Could you check a few things on this model? Use its own coordinates, in mm. Face numbers are marked on the shaded views. A direction names the side the tool comes from. Give positions to 0.01 mm unless a question says otherwise; leave off trailing zeros. Order: outer loops, then holes, each group sorted by start corner. A loop starts at its lowest first (then second) coordinate and runs counter-clockwise, first axis right, second up.
from build123d import *

# Parameters (mm, degrees)
F1_DEPTH  = 12.6
F2_R      = 6
F3_DEPTH  = 16
F4_R      = 3.85
F5_DEPTH  = 5.8
F6_R      = 4.35
F7_DEPTH  = 3.6
F8_R      = 2
F9_R      = 1.5
F10_W     = 1
F10_H     = 5
F11_DEPTH = 5
F12_R     = 1.2
F13_DEPTH = 10.501


with BuildPart() as f1:
    # F0 (on Top) → F1 (new body)
    with BuildSketch(Plane.XY):
        with BuildLine():
            Line((-6.15, -6.5), (12.65, -6.5))
            Line((12.65, -6.5), (12.65, 6.5))
            Line((12.65, 6.5), (-6.15, 6.5))
            ThreePointArc((-6.15, 6.5), (-10.746194, 4.596194), (-12.65, 0))
            ThreePointArc((-12.65, 0), (-10.746194, -4.596194), (-6.15, -6.5))
        make_face()
    extrude(amount=-F1_DEPTH)

    # F2 (on Top) → F3 (join)
    with BuildSketch(Plane.XY):
        Circle(F2_R)
    extrude(amount=F3_DEPTH)

    # F4 (on face) → F5 (join)
    with BuildSketch(Plane.XY.offset(16)):
        Circle(F4_R)
    extrude(amount=F5_DEPTH)

    # F6 (on face) → F7 (join)
    with BuildSketch(Plane.XY.offset(21.8)):
        Circle(F6_R)
    extrude(amount=F7_DEPTH)

    # F8
    f8_edges = [f1.edges().sort_by_distance(p)[0] for p in [
        (-4.35, 0, 25.4),
    ]]
    fillet(f8_edges, radius=F8_R)

    # F9
    f9_edges = [f1.edges().sort_by_distance(p)[0] for p in [
        (3.25, -6.5, -12.6),
        (12.65, 0, -12.6),
        (3.25, 6.5, -12.6),
        (-12.65, 0, -12.6),
    ]]
    fillet(f9_edges, radius=F9_R)

    # F10 (on face) → F11 (join)
    with BuildSketch(Plane.YZ.offset(12.65)):
        with Locations((-3.5, -3.5)):
            Rectangle(F10_W, F10_H)
        with Locations((3.5, -3.5)):
            Rectangle(F10_W, F10_H)
    extrude(amount=F11_DEPTH)

    # F12 (on face) → F13 (cut, through all)
    with BuildSketch(Plane.XZ.offset(4)):
        with Locations((15.15, -3.5)):
            Circle(F12_R)
        with BuildLine():
            Line((12.65, -1), (12.65, -2))
            ThreePointArc((12.65, -2), (13.079724, -1.904888), (13.45, -1.66697))
            ThreePointArc((13.45, -1.66697), (14.236922, -1.172708), (15.15, -1))
            Line((15.15, -1), (12.65, -1))
        make_face()
        with BuildLine():
            ThreePointArc((17.65, -3.5), (16.917767, -5.267767), (15.15, -6))
            Line((15.15, -6), (17.65, -6))
            Line((17.65, -6), (17.65, -3.5))
        make_face()
        with BuildLine():
            ThreePointArc((15.15, -1), (16.917767, -1.732233), (17.65, -3.5))
            Line((17.65, -3.5), (17.65, -1))
            Line((17.65, -1), (15.15, -1))
        make_face()
        with BuildLine():
            ThreePointArc((15.15, -6), (14.236922, -5.827292), (13.45, -5.33303))
            ThreePointArc((13.45, -5.33303), (13.079724, -5.095112), (12.65, -5))
            Line((12.65, -5), (12.65, -6))
            Line((12.65, -6), (15.15, -6))
        make_face()
    extrude(amount=-F13_DEPTH, mode=Mode.SUBTRACT)


solid = f1.part
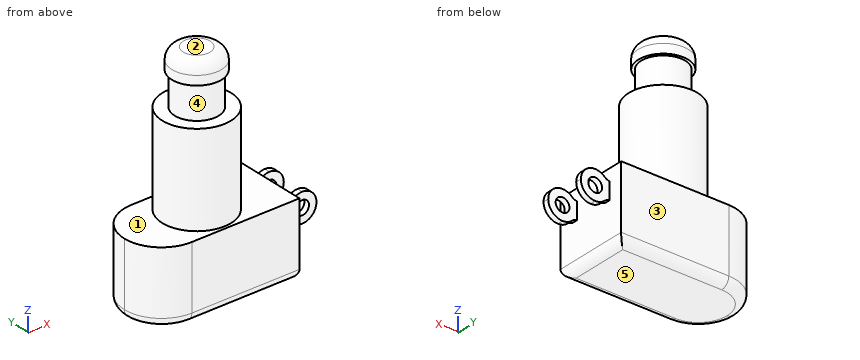
Item 1: For the marked faces 1 and 2, which set-ups out of +Z, -Z, +X, -X, +Y, -Y let a thin tool reach every point of the face, with its end or its side?
Findings:
face 1: +Z
face 2: +Z, +X, -X, +Y, -Y
Item 2: Please list where these lines run through material, in increasing order: line 1 along Z through (x, y) = (15.15, 3.45); line 2 along Y through (x, z) = (13, -3.5); line 3 along Z through (x, y) = (7.5, -3.75).
Findings:
line 1: z = -6 to -4.7, -2.3 to -1
line 2: y = -4 to -3, 3 to 4
line 3: z = -12.6 to 0
Item 3: We'd pull the mould along Z, two halves only. Please class the marked faces 3, 4 and 5: +Z half, -Z half, draft (parallel to the pull), parting line (faces both ways), or undercut.
Findings:
face 3: draft
face 4: undercut
face 5: -Z half
Item 4: Imagine slicing it at B-B on z = -9. List the corners of the cut face in (x, y) for me, then the cut area to 3 significant figures.
Findings:
outline: (-6.15, -6.5) - (12.65, -6.5) - (12.65, 6.5) - (-6.15, 6.5) arc R6.5 ccw to start
area: 311 mm2
Item 5: Imagine slicing it at A-A on x = 0. List the corners of the cut face in (y, z) for me.
Findings:
outline: (-6.5, -11.1) arc R1.5 ccw to (-5, -12.6) - (5, -12.6) arc R1.5 ccw to (6.5, -11.1) - (6.5, 0) - (6, 0) - (6, 16) - (3.85, 16) - (3.85, 21.8) - (4.35, 21.8) - (4.35, 23.4) arc R2 ccw to (2.35, 25.4) - (-2.35, 25.4) arc R2 ccw to (-4.35, 23.4) - (-4.35, 21.8) - (-3.85, 21.8) - (-3.85, 16) - (-6, 16) - (-6, 0) - (-6.5, 0) - close
Item 6: Imagine slicing it at C-C on z = 15. List the corners of the cut face in (x, y) for me, then the cut area to 3 significant figures.
Findings:
outline: circle Ø12 at (0, 0)
area: 113 mm2
Item 7: For pin 1 (4 mm diameter, centred on x = 15.15, z = -3.5, fed in from -Y); pin 2 (1 mm diameter, centred on y = 5, z = -4, fed in from +X); pin 3 (3 mm diameter, centred on x = 6.5, z = 7, fed in from +Y), each with a flat end and sliding along its axis, tell me the tip position at first contact or that it passes through.
Findings:
pin 1: stops at y = -4
pin 2: stops at x = 12.65
pin 3: stops at y = 3.32
Item 8: Imagine slicing it at D-D on z = 21. List the corners of the cut face in (x, y) for me.
Findings:
outline: circle Ø7.7 at (0, 0)
